Geometry check sheet. Reference: the model listing, model coordinates, mm. A direction names the side the tool comes from. Give positions to 0.01 mm unless a question says otherwise; leave off trailing zeros. Write each loop counter-clockwise with the first axis right and the second up, starting at its lowest first coordinate (ties: lowest second). Pieces come first, ordered by that corner, then holes.
(1) Mould release check, pull along X, two halves, no side actions. Record for faces 1 (the flat face through (11, 20, 0)), 2 (the flat face through (10.5, 19, 725)), 3 (the flat face through (-12.5, 18, 725)): +X half, -X half, draft (parallel to the pull), parting line (faces both ways), or undercut.
(2) Depth check by flat-ended pin: P1, Ø5, axis at y = 22.5, z = 385.5, coming from the +X side; P2, Ø10, axis at x = 2, y = 43.5, coming from the -Z side; P3, Ø3.5, axis at x = 20, y = 28, coming from the +Z side. Enter the tip coordinate at first touch or a pass-through.
(3) Cross-section at A-A (y = 16.5). Record the boundary of the cut face in (x, z).
(4) Cross-section at B-B (z = 687). Record the boundary of the cut face in (x, y), and give its area (3 significant figures).
(5) Tool access check on faces 4 (the flat face through (24, 30, 570)), 5 (the flat face through (24, 27, 1002)), 6 (the flat face through (11, 20, 1470)), 7 (the flat face through (-10.5, 18, 725)). Record the directions out of +Z, -Z, +X, -X, +Y, -Y that give a thin tool (end or side, any length) a straight path to the whole face; none if there is none.
(6) Thickness scan on line 1 along Z through (x, y) = (13, 28); line 2 along X through (y, z) = (56.1, 172.55); line 3 along Y through (x, z) = (10, 305). Record the ranges inside material, lowest first.
```python
from build123d import *

# Parameters (mm, degrees)
EXTRUDE_THIN1_DEPTH  = 1470
SKETCH2_R            = 4
BOSS_EXTRUDE1_DEPTH  = 3
SKETCH3_W            = 16
SKETCH3_H            = 16
EXTRUDE_THIN2_DEPTH  = 60
M3_CLEARANCE_HOLE1_D = 3.2
LPATTERN1_COUNT      = 4
LPATTERN1_PITCH      = 300


with BuildPart() as part:
    # Sketch1 → Extrude-Thin1 (new body)
    with BuildSketch(Plane.XY):
        with BuildLine():
            Line((-9.5, 37), (9.5, 37))
            ThreePointArc((9.5, 37), (11.621320344, 36.121320344), (12.5, 34))
            Line((12.5, 34), (12.5, 3))
            ThreePointArc((12.5, 3), (11.621320344, 0.878679656), (9.5, 0))
            Line((9.5, 0), (-9.5, 0))
            ThreePointArc((-9.5, 0), (-11.621320344, 0.878679656), (-12.5, 3))
            Line((-12.5, 3), (-12.5, 34))
            ThreePointArc((-12.5, 34), (-11.621320344, 36.121320344), (-9.5, 37))
        make_face()
        with BuildLine():
            Line((-9.5, 35), (9.5, 35))
            ThreePointArc((9.5, 35), (10.207106781, 34.707106781), (10.5, 34))
            Line((10.5, 34), (10.5, 3))
            ThreePointArc((10.5, 3), (10.207106781, 2.292893219), (9.5, 2))
            Line((9.5, 2), (-9.5, 2))
            ThreePointArc((-9.5, 2), (-10.207106781, 2.292893219), (-10.5, 3))
            Line((-10.5, 3), (-10.5, 34))
            ThreePointArc((-10.5, 34), (-10.207106781, 34.707106781), (-9.5, 35))
        make_face(mode=Mode.SUBTRACT)
    extrude(amount=EXTRUDE_THIN1_DEPTH)

    # Sketch2 → Boss-Extrude1 (add)
    with BuildSketch(Plane(origin=(0, 27, 0), x_dir=(1, 0, 0), z_dir=(0, 1, 0))):
        with BuildLine():
            Line((29.5, -103), (12.5, -103))
            Line((12.5, -103), (12.5, -127))
            Line((12.5, -127), (29.5, -127))
            ThreePointArc((29.5, -127), (41.5, -115), (29.5, -103))
        make_face()
        with Locations((29.5, -115)):
            Circle(SKETCH2_R, mode=Mode.SUBTRACT)
        with BuildLine():
            Line((29.5, -558), (12.5, -558))
            Line((12.5, -558), (12.5, -582))
            Line((12.5, -582), (29.5, -582))
            ThreePointArc((29.5, -582), (41.5, -570), (29.5, -558))
        make_face()
        with Locations((29.5, -570)):
            Circle(SKETCH2_R, mode=Mode.SUBTRACT)
        with BuildLine():
            Line((29.5, -990), (12.5, -990))
            Line((12.5, -990), (12.5, -1014))
            Line((12.5, -1014), (29.5, -1014))
            ThreePointArc((29.5, -1014), (41.5, -1002), (29.5, -990))
        make_face()
        with Locations((29.5, -1002)):
            Circle(SKETCH2_R, mode=Mode.SUBTRACT)
    extrude(amount=BOSS_EXTRUDE1_DEPTH)

    # Sketch3 → Extrude-Thin2 (add)
    with BuildSketch(Plane(origin=(0, 0, 150), x_dir=(-1, 0, 0), z_dir=(0, 0, -1))):
        with BuildLine():
            Line((10, 55), (10, 39))
            ThreePointArc((10, 39), (9.414213562, 37.585786438), (8, 37))
            Line((8, 37), (-8, 37))
            ThreePointArc((-8, 37), (-9.414213562, 37.585786438), (-10, 39))
            Line((-10, 39), (-10, 55))
            ThreePointArc((-10, 55), (-9.414213562, 56.414213562), (-8, 57))
            Line((-8, 57), (8, 57))
            ThreePointArc((8, 57), (9.414213562, 56.414213562), (10, 55))
        make_face()
        with Locations((0, 47)):
            Rectangle(SKETCH3_W, SKETCH3_H, mode=Mode.SUBTRACT)
    extrude_thin2 = extrude(amount=-EXTRUDE_THIN2_DEPTH)

    # M3 Clearance Hole1 (through all)
    with Locations(Plane(origin=(0, 57, 0), x_dir=(1, 0, 0), z_dir=(0, 1, 0))):
        with Locations((0, -187.45), (0, -172.55)):
            m3_clearance_hole1 = Hole(M3_CLEARANCE_HOLE1_D / 2)

    # LPattern1: Extrude-Thin2, M3 Clearance Hole1 ×4
    with Locations(*[(0, 0, i * LPATTERN1_PITCH) for i in range(1, LPATTERN1_COUNT)]):
        add(extrude_thin2)
        add(m3_clearance_hole1, mode=Mode.SUBTRACT)


solid = part.part
```
Reply:
1. face 1: draft
1. face 2: undercut
1. face 3: -X half
2. P1: stops at x = 12.5
2. P2: stops at z = 150
2. P3: stops at z = 1014
3. outline: (-12.5, 0) - (-10.5, 0) - (-10.5, 1470) - (-12.5, 1470) - close; (10.5, 0) - (12.5, 0) - (12.5, 1470) - (10.5, 1470) - close
4. outline: (-12.5, 3) arc R3 ccw to (-9.5, 0) - (9.5, 0) arc R3 ccw to (12.5, 3) - (12.5, 34) arc R3 ccw to (9.5, 37) - (-9.5, 37) arc R3 ccw to (-12.5, 34) - close; hole (-10.5, 3) arc R1 ccw to (-9.5, 2) - (9.5, 2) arc R1 ccw to (10.5, 3) - (10.5, 34) arc R1 ccw to (9.5, 35) - (-9.5, 35) arc R1 ccw to (-10.5, 34) - close
4. area: 225 mm2
5. face 4: +Z, -Z, +X, +Y
5. face 5: +Z, -Z, +X, -Y
5. face 6: +Z, +X, -X, +Y, -Y
5. face 7: +Z, -Z
6. line 1: z = 103 to 127, 558 to 582, 990 to 1014
6. line 2: x = -9.67 to -1.6, 1.6 to 9.67
6. line 3: y = 0.04 to 2.13, 34.87 to 36.96
